```python
from build123d import *

# Parameters (mm, degrees)
REVOLVE_1_ANGLE     = 180
SKETCH_2_W          = 82.604360497
SKETCH_2_H          = 69.359352877
CUT_EXTRUDE_1_DEPTH = 1.5
SKETCH_3_R          = 1.6
SKETCH_3_W          = 3
SKETCH_3_H          = 43
EXTRUDE_1_DEPTH     = 5
FILLET_1_R          = 8


with BuildPart() as part:
    # 草图1 → 旋转1 (revolve)
    with BuildSketch(Plane.XY):
        Polygon((22.5, 29.467251478), (21.5, 29.467251478), (21.5, 39.467251478), (30, 39.467251478), (30, -3.532748522), (21.5, -3.532748522), (21.5, 4.467251478), (22.5, 4.467251478), (22.5, 9.467251478), (25, 9.467251478), (25, 14.467251478), (22.5, 14.467251478), (22.5, 19.467251478), (25, 19.467251478), (25, 24.467251478), (22.5, 24.467251478), align=None)
    revolve(axis=Axis((0, 80.879290808, 0), (0, -1, 0)), revolution_arc=REVOLVE_1_ANGLE)

    # 草图2 → 切除-拉伸1 (cut)
    with BuildSketch(Plane(origin=(0, 0, 0), x_dir=(-1, 0, 0), z_dir=(0, 0, -1))):
        with Locations((1.112176212, 17.562823765)):
            Rectangle(SKETCH_2_W, SKETCH_2_H)
    extrude(amount=-CUT_EXTRUDE_1_DEPTH, mode=Mode.SUBTRACT)

    # 草图3 → 凸台-拉伸1 (add)
    # profile 1 of 3: a face of its own
    with BuildSketch(Plane(origin=(0, 0, 1.5), x_dir=(-1, 0, 0), z_dir=(0, 0, -1))):
        with BuildLine():
            ThreePointArc((49.962476533, 1.467251478), (48.498010439, -2.068282428), (44.962476533, -3.532748522))
            Line((44.962476533, -3.532748522), (29.962476533, -3.532748522))
            Line((29.962476533, -3.532748522), (29.962476533, 39.467251478))
            Line((29.962476533, 39.467251478), (44.962476533, 39.467251478))
            ThreePointArc((44.962476533, 39.467251478), (48.498010439, 38.002785384), (49.962476533, 34.467251478))
            Line((49.962476533, 34.467251478), (49.962476533, 1.467251478))
        make_face()
        with Locations((41.962476533, 17.967251478)):
            Circle(SKETCH_3_R, mode=Mode.SUBTRACT)
        with Locations((41.962476533, 4.967251478)):
            Circle(SKETCH_3_R, mode=Mode.SUBTRACT)
        with Locations((41.962476533, 30.967251478)):
            Circle(SKETCH_3_R, mode=Mode.SUBTRACT)
    # profile 2 of 3: a face of its own
    with BuildSketch(Plane(origin=(0, 0, 1.5), x_dir=(-1, 0, 0), z_dir=(0, 0, -1))):
        with Locations((28.462476533, 17.967251478)):
            Rectangle(SKETCH_3_W, SKETCH_3_H)
    # profile 3 of 3: a face of its own
    with BuildSketch(Plane(origin=(0, 0, 1.5), x_dir=(-1, 0, 0), z_dir=(0, 0, -1))):
        with BuildLine():
            Line((-29.962476533, 39.467251478), (-44.962476533, 39.467251478))
            ThreePointArc((-44.962476533, 39.467251478), (-48.498010439, 38.002785384), (-49.962476533, 34.467251478))
            Line((-49.962476533, 34.467251478), (-49.962476533, 1.467251478))
            ThreePointArc((-49.962476533, 1.467251478), (-48.498010439, -2.068282428), (-44.962476533, -3.532748522))
            Line((-44.962476533, -3.532748522), (-29.962476533, -3.532748522))
            Line((-29.962476533, -3.532748522), (-26.962476533, -3.532748522))
            Line((-26.962476533, -3.532748522), (-26.962476533, 39.467251478))
            Line((-26.962476533, 39.467251478), (-29.962476533, 39.467251478))
        make_face()
        with Locations((-41.962476533, 30.967251478)):
            Circle(SKETCH_3_R, mode=Mode.SUBTRACT)
        with Locations((-41.962476533, 17.967251478)):
            Circle(SKETCH_3_R, mode=Mode.SUBTRACT)
        with Locations((-41.962476533, 4.967251478)):
            Circle(SKETCH_3_R, mode=Mode.SUBTRACT)
    extrude(amount=-EXTRUDE_1_DEPTH)

    # 圆角1
    fillet_1_edges = [part.edges().sort_by_distance(p)[0] for p in [
        (-29.287369291, 17.967251478, 6.5),
        (29.287369291, 17.967251478, 6.5),
    ]]
    fillet(fillet_1_edges, radius=FILLET_1_R)


solid = part.part
```
The model under review builds one solid part; all positions refer to its coordinate system, in mm. A direction names the side the tool comes from. Give positions to 0.01 mm unless a question says otherwise; leave off trailing zeros. Write each loop counter-clockwise with the first axis right and the second up, starting at its lowest first coordinate (ties: lowest second). Pieces come first, ordered by that corner, then holes. Notation, with made-up numbers: (-8, 23.25) -> (35, 23.25) arc R17 ccw to (35, 45.25) -> close; hole circle Ø7 at (-27.75, 82.25). An arc over 180 degrees is marked (long way). Answer in a Markdown table with one row per item.
1) Tool access review of faces 5 (the cylindrical face through (43.14, 6.05, 3.96)), 6 (the flat face through (-44, 18, 6.5)), 7 (the flat face through (0, 24.467, 23)): name each direction out of +Z, -Z, +X, -X, +Y, -Y from which nothing blocks a thin tool from reaching the whole face with its end or side.
Worked answers:
| item | result |
|---|---|
| face 5 | +Z, -Z |
| face 6 | +Z, -X, +Y, -Y |
| face 7 | -Z |
2) Add section B-B on y = 22. State the section outline as (x, z) points, plus the area to 3 significant figures.
Worked answers:
| item | result |
|---|---|
| outline | (-49.96, 1.5) -> (-24.95, 1.5) arc R25 cw to (24.95, 1.5) -> (49.96, 1.5) -> (49.96, 6.5) -> (35.12, 6.5) arc R8 cw to (27.73, 11.45) arc R30 ccw to (-27.73, 11.45) arc R8 cw to (-35.12, 6.5) -> (-49.96, 6.5) -> close |
| area | 631 mm² |
3) Add section D-D on z = 5. Count the separate pieces of the cut face and the enclosed holes in it, plus the area to 3 significant figures.
Worked answers:
| item | result |
|---|---|
| separate pieces | 2 |
| enclosed holes | 6 |
| area | 2,330 mm² |
4) Clearance check with flat-ended pins moving along their axes: P1, Ø12, axis at x = 3, z = 11.5, coming from the +Y side; P2, Ø5, axis at x = -41.96, y = 30.97, coming from the +Z side; P3, Ø4, axis at y = 6, z = 17, coming from the -X side; P4, Ø6, axis at y = 12, z = 20.5, coming from the +X side. State where each tip first meets the part, or that it passes through.
Worked answers:
| item | result |
|---|---|
| P1 | through |
| P2 | z = 6.5 |
| P3 | x = -25.98 |
| P4 | x = 24.37 |
5) Add section A-A on x = 0. State the section outline as (y, z) points, plus the area to 4 significant figures.
Worked answers:
| item | result |
|---|---|
| outline | (-3.53, 21.5) -> (4.47, 21.5) -> (4.47, 22.5) -> (9.47, 22.5) -> (9.47, 25) -> (14.47, 25) -> (14.47, 22.5) -> (19.47, 22.5) -> (19.47, 25) -> (24.47, 25) -> (24.47, 22.5) -> (29.47, 22.5) -> (29.47, 21.5) -> (39.47, 21.5) -> (39.47, 30) -> (-3.53, 30) -> close |
| area | 315.5 mm² |
6) Mouldability with a two-part tool opening along Y and no side actions: class faces 1 (the cylindrical face through (-48.537, -2.029, 3.965)), 2 (the cylindrical face through (0.452, 0.523, 21.495)), 3 (the cylindrical face through (43.23, 29.99, 3.96)), 4 (the cylindrical face through (-42.701, 29.548, 3.965)) as +Y half, -Y half, draft (parallel to the pull), parting line (faces both ways), or undercut.
Worked answers:
| item | result |
|---|---|
| face 1 | -Y half |
| face 2 | draft |
| face 3 | undercut |
| face 4 | undercut |
7) For L1, parallel to X at y = 14.5, z = 11.5; L2, parallel to X at y = 13, z = 6; L3, parallel to Y at x = -21, z = 7.5, list the stretches that pass through material, from the lowest coordinate up. Write a range as [from, to].
Worked answers:
| item | result |
|---|---|
| L1 | [-27.71, -19.34], [19.34, 27.71] |
| L2 | [-49.96, -24.27], [24.27, 49.96] |
| L3 | [-3.53, 4.47], [29.47, 39.47] |
